from build123d import *

# Parameters (mm, degrees)
SKETCH1_W           = 85
SKETCH1_H           = 24
BOSS_EXTRUDE1_DEPTH = 3
SKETCH2_W           = 85
SKETCH2_H           = 17.5
BOSS_EXTRUDE2_DEPTH = 3
SKETCH3_W           = 85
SKETCH3_H           = 3
BOSS_EXTRUDE3_DEPTH = 3.5
SKETCH4_R           = 1.65
CUT_EXTRUDE1_DEPTH  = 3
SKETCH5_R           = 1.6
CUT_EXTRUDE2_DEPTH  = 3
SKETCH6_W           = 85
SKETCH6_H           = 27
BOSS_EXTRUDE4_DEPTH = 3
SKETCH7_W           = 85
SKETCH7_H           = 21
CUT_EXTRUDE3_DEPTH  = 4
BOSS_EXTRUDE5_DEPTH = 4
FILLET4_R           = 0.5
SKETCH9_W           = 7
SKETCH9_H           = 10
BOSS_EXTRUDE6_DEPTH = 8
CHAMFER1_SIZE       = 0.7
CHAMFER2_SIZE       = 0.5


with BuildPart() as part:
    # Sketch1 → Boss-Extrude1 (new body)
    with BuildSketch(Plane(origin=(0, 0, 0), x_dir=(1, 0, 0), z_dir=(0, 1, 0))):
        Rectangle(SKETCH1_W, SKETCH1_H)
    extrude(amount=BOSS_EXTRUDE1_DEPTH)

    # Sketch2 → Boss-Extrude2 (add)
    with BuildSketch(Plane.XY.offset(12)):
        with Locations((0, 8.75)):
            Rectangle(SKETCH2_W, SKETCH2_H)
    extrude(amount=BOSS_EXTRUDE2_DEPTH)

    # Sketch3 → Boss-Extrude3 (add)
    with BuildSketch(Plane(origin=(0, 3, 0), x_dir=(1, 0, 0), z_dir=(0, 1, 0))):
        with Locations((0, 10.5)):
            Rectangle(SKETCH3_W, SKETCH3_H)
    extrude(amount=BOSS_EXTRUDE3_DEPTH)

    # Sketch4 → Cut-Extrude1 (cut)
    with BuildSketch(Plane.XY.offset(15)):
        with Locations((-39, 11.5)):
            Circle(SKETCH4_R)
        with Locations((32, 11.5)):
            Circle(SKETCH4_R)
    extrude(amount=-CUT_EXTRUDE1_DEPTH, mode=Mode.SUBTRACT)

    # Sketch5 → Cut-Extrude2 (cut)
    with BuildSketch(Plane(origin=(0, 0, -12), x_dir=(-1, 0, 0), z_dir=(0, 0, -1))):
        with Locations((39, 3.5)):
            Circle(SKETCH5_R)
        with Locations((-19.1, 3.5)):
            Circle(SKETCH5_R)
    extrude(amount=-CUT_EXTRUDE2_DEPTH, mode=Mode.SUBTRACT)

    # Sketch6 → Boss-Extrude4 (add)
    with BuildSketch(Plane.XZ):
        with Locations((0, 1.5)):
            Rectangle(SKETCH6_W, SKETCH6_H)
    extrude(amount=BOSS_EXTRUDE4_DEPTH)

    # Sketch7 → Cut-Extrude3 (cut)
    with BuildSketch(Plane(origin=(0, 3, 0), x_dir=(1, 0, 0), z_dir=(0, 1, 0))):
        with Locations((0, -1.5)):
            Rectangle(SKETCH7_W, SKETCH7_H)
    extrude(amount=-CUT_EXTRUDE3_DEPTH, mode=Mode.SUBTRACT)

    # Sketch8 → Boss-Extrude5 (add)
    with BuildSketch(Plane.ZY.offset(42.5)):
        Polygon((-12, 6.5), (-9, 6.5), (-9, -1), (12, -1), (12, 17.5), (15, 17.5), (15, -3), (-12, -3), align=None)
    extrude(amount=BOSS_EXTRUDE5_DEPTH)

    # Fillet4
    fillet4_edges = [part.edges().sort_by_distance(p)[0] for p in [
        (42.5, 8.25, 12),
        (-2, 17.5, 12),
        (42.5, 17.5, 13.5),
        (42.5, 7.25, 15),
        (-2, 17.5, 15),
        (42.5, 2.75, -9),
        (-2, 6.5, -9),
        (42.5, 6.5, -10.5),
        (-2, 6.5, -12),
        (-37.4, 3.5, -12),
        (20.7, 3.5, -12),
        (-2, -3, -12),
        (-2, -1, -9),
        (42.5, -1, 1.5),
        (-2, -1, 12),
        (42.5, 1.75, -12),
        (-46.5, 1.75, -12),
        (-46.5, 7.25, 15),
        (-46.5, 8.25, 12),
        (-46.5, -1, 1.5),
        (-46.5, 2.75, -9),
        (-46.5, 6.5, -10.5),
    ]]
    fillet(fillet4_edges, radius=FILLET4_R)

    # Sketch9 → Boss-Extrude6 (add)
    with BuildSketch(Plane.XZ.offset(3)):
        with Locations((0, 1.5)):
            Rectangle(SKETCH9_W, SKETCH9_H)
    extrude(amount=BOSS_EXTRUDE6_DEPTH)

    # Chamfer1
    chamfer1_edges = [part.edges().sort_by_distance(p)[0] for p in [
        (3.5, -11, 1.5),
        (0, -11, 6.5),
        (-3.5, -11, 1.5),
        (0, -11, -3.5),
    ]]
    chamfer(chamfer1_edges, length=CHAMFER1_SIZE)

    # Chamfer2
    chamfer2_edges = [part.edges().sort_by_distance(p)[0] for p in [
        (3.5, -6.65, -3.5),
        (-3.5, -6.65, -3.5),
        (-3.5, -6.65, 6.5),
        (3.5, -6.65, 6.5),
    ]]
    chamfer(chamfer2_edges, length=CHAMFER2_SIZE)


solid = part.part
The listing builds one solid part. Answer for the finished solid, in the listing's coordinates (mm). A direction names the side the tool comes from. Give positions to 0.01 mm unless a question says otherwise; leave off trailing zeros. Order: outer loops, then holes, each group sorted by start corner. A loop starts at its lowest first (then second) coordinate and runs counter-clockwise, first axis right, second up. Notation, with made-up numbers: (40, 23.25) - (99, 23.25) arc R19 cw to (99, 31.25) - close; hole circle Ø6 at (-8.75, -16.5). An arc over 180 degrees is marked (long way). One line per item, written item: value. Start each with the question number.
1) The mould has two halves that part along Y. Classify faces 1 (the face through (-1, -3, 8)), 2 (the face through (-3.5, -7, 1)), 3 (the face through (17.574, 3.981, -10.268)), 4 (the face through (-2, 17.5, 13)): released by +Y, released by -Y, zero draft, split by the parting line, or undercut.
2) A cutting plane is placed at B-B on x = 32. Give the vertices of the cut face in (y, z), then the cut area to 3 significant figures.
3) A cutting plane is placed at C-C on x = -39. Give the vertices of the cut face in (y, z).
4) A cutting plane is placed at A-A on y = 11.5. Give the vertices of the cut face in (x, z).
5) A tool of negligible diameter and unlimited length cuts with its end or side. For faces 5 (the face through (-1, -1, 1)), 6 (the face through (3.5, -7, 1)), 7 (the face through (-1, 6.5, -11)), 8 (the face through (0, -7, 6.5)), 9 (the face through (-37.82, 4.58, -10.27)), from which of +Z, -Z, +X, -X, +Y, -Y can it reach the whole face along a straight path? Write none if from no direction.
6) Given pin 1 Ø10 at (x, z) = (13.5, -1.5) entering from +Y; pin 2 Ø2 at (x, z) = (-20.5, 1.5) entering from -Y; pin 3 Ø3.5 at (x, y) = (19.1, 3.5) entering from -Z; pin 4 Ø4 at (y, z) = (9, 8.5) entering from +X (3 decimals), each flat-ended and moving along its own axis, determine where each tip first touches the part or whether it passes through.
7) Find the intervals of material crossed by L1, parallel to Y at x = -39, z = 13.8; L2, parallel to Y at x = -39, z = -10.3; L3, parallel to Z at x = 23.5, y = 3.5, in increasing order.
8) A cutting plane is placed at D-D on z = 0.5. Give the vertices of the cut face in (x, y).
Answer sheet:
1. face 1: released by -Y
1. face 2: zero draft
1. face 3: undercut
1. face 4: released by +Y
2. outline: (-3, -11.5) arc R0.5 ccw to (-2.5, -12) - (6, -12) arc R0.5 ccw to (6.5, -11.5) - (6.5, -9.5) arc R0.5 ccw to (6, -9) - (-0.5, -9) arc R0.5 cw to (-1, -8.5) - (-1, 11.5) arc R0.5 cw to (-0.5, 12) - (9.85, 12) - (9.85, 15) - (-3, 15) - close; (13.15, 12) - (17, 12) arc R0.5 ccw to (17.5, 12.5) - (17.5, 14.5) arc R0.5 ccw to (17, 15) - (13.15, 15) - close
2. area: 122 mm2
3. outline: (-3, -11.5) arc R0.5 ccw to (-2.5, -12) - (1.4, -12) arc R0.5 ccw to (1.9, -11.5) - (1.9, -9) - (-0.5, -9) arc R0.5 cw to (-1, -8.5) - (-1, 11.5) arc R0.5 cw to (-0.5, 12) - (9.85, 12) - (9.85, 15) - (-3, 15) - close; (5.1, -11.5) arc R0.5 ccw to (5.6, -12) - (6, -12) arc R0.5 ccw to (6.5, -11.5) - (6.5, -9.5) arc R0.5 ccw to (6, -9) - (5.1, -9) - close; (13.15, 12) - (17, 12) arc R0.5 ccw to (17.5, 12.5) - (17.5, 14.5) arc R0.5 ccw to (17, 15) - (13.15, 15) - close
4. outline: (-46.5, 12.5) arc R0.5 ccw to (-46, 12) - (-40.65, 12) - (-40.65, 15) - (-46, 15) arc R0.5 ccw to (-46.5, 14.5) - close; (-37.35, 12) - (30.35, 12) - (30.35, 15) - (-37.35, 15) - close; (33.65, 12) - (42, 12) arc R0.5 ccw to (42.5, 12.5) - (42.5, 14.5) arc R0.5 ccw to (42, 15) - (33.65, 15) - close
5. face 5: +X, -X, +Y
5. face 6: +Z, -Z, +X, -Y
5. face 7: -Z, +X, -X, +Y
5. face 8: +Z, +X, -X, -Y
5. face 9: -Z
6. pin 1: stops at y = -1
6. pin 2: stops at y = -3
6. pin 3: stops at z = -11.86
6. pin 4: passes through
7. L1: y = -3 to 9.85, 13.15 to 17.5
7. L2: y = -3 to 1.9, 5.1 to 6.5
7. L3: z = -12 to -9, 12 to 15
8. outline: (-46.5, -3) - (-3.5, -3) - (-3.5, -10.3) - (-2.8, -11) - (2.8, -11) - (3.5, -10.3) - (3.5, -3) - (42.5, -3) - (42.5, -1.5) arc R0.5 ccw to (42, -1) - (-46, -1) arc R0.5 ccw to (-46.5, -1.5) - close
